Autodesk Inventor part; units mm, degrees
ref_plane "YZ Plane" through (0, 0, 0) normal (1, 0, 0) x (0, 1, 0)
ref_plane "XZ Plane" through (0, 0, 0) normal (0, 1, 0) x (-1, 0, 0)
ref_plane "XY Plane" through (0, 0, 0) normal (0, 0, 1) x (1, 0, 0)
sketch "Sketch1" plane through (0, 0, 0) normal (0, 1, 0) x (-1, 0, 0)
  circle A0 centre (0, 0) radius 17.1346
extrude "Extrusion1" add sketch "Sketch1" along normal blind 10
sketch "Sketch2" plane through (0, 0, 0) normal (0, -1, 0) x (1, 0, 0)
  circle A0 centre (0, 0) radius 14.2353
extrude "Extrusion2" add sketch "Sketch2" along normal blind 5
chamfer "Chamfer1" distance 2 angle 45 1 edges at (-14.2353, -5, 0)
properties part number "Tapon externo"
For this review, take the finished solid that the model builds, in its own axes (mm). A direction names the side the tool comes from. Coordinates: 2 decimals unless noted, no trailing zeros. Order: outer loops, then holes, each group sorted by start corner. A loop starts at its lowest first (then second) coordinate and runs counter-clockwise, first axis right, second up. Notation, with made-up numbers: (46.5, 25.25) -> (57.5, 25.25) arc R27 ccw to (57.5, 43.25) -> close; hole circle Ø7 at (21, -9.5). An arc over 180 degrees is marked (long way). Use CSV: the item, a comma, the result in double quotes. Start each with the question number.
Item 1: For faces 1 (the face through (4, 0, 14)), 2 (the face through (-16.343, 4.93, -5.147)), list the 3-axis set-ups (+Z, -Z, +X, -X, +Y, -Y) from which the entire face can be reached by the end or side of a thin tool; tool diameter is ignored.
Item 2: We need section A-A, the plane x = 0. Give the boundary of the cut face in (y, z).
Item 3: We need section D-D, the plane y = -2. Give the boundary of the cut face in (x, z), then the cut area to 3 significant figures.
Item 4: Insertion check: pin 1 (5 mm diameter, centred on y = 4.5, z = -11, fed in from -X); pin 2 (3 mm diameter, centred on y = 3, z = 12.5, fed in from +X); pin 3 (1 mm diameter, centred on y = 2, z = 9.5, fed in from -X). Each pin has a flat end and moves straight along its axis. Give the tip position at first contact, or say it passes through.
Item 5: We need section B-B, the plane z = 0. Give the boundary of the cut face in (x, y), then the cut area to 3 significant figures.
Item 6: We need section C-C, the plane y = 5.5. Give the boundary of the cut face in (x, z), then the cut area to 3 significant figures.
Item 7: Wall thickness on probe 1 along Y at (x, z) = (12.5, -11.5); probe 2 along Z at (x, y) = (-14, 6.75); probe 3 along Z at (x, y) = (15, 7): over which ranges is each line inside the solid? List them lowest first.
Derived:
1,face 1,"-Y"
1,face 2,"+Y, -Y"
2,outline,"(-5, -12.24) -> (-3, -14.24) -> (0, -14.24) -> (0, -17.13) -> (10, -17.13) -> (10, 17.13) -> (0, 17.13) -> (0, 14.24) -> (-3, 14.24) -> (-5, 12.24) -> close"
3,outline,"circle Ø28.47 at (0, 0)"
3,area,"637 mm^2"
4,pin 1,"stops at x = -14.88"
4,pin 2,"stops at x = 13.14"
4,pin 3,"stops at x = -14.58"
5,outline,"(-17.13, 0) -> (-14.24, 0) -> (-14.24, -3) -> (-12.24, -5) -> (12.24, -5) -> (14.24, -3) -> (14.24, 0) -> (17.13, 0) -> (17.13, 10) -> (-17.13, 10) -> close"
5,area,"481 mm^2"
6,outline,"circle Ø34.27 at (0, 0)"
6,area,"922 mm^2"
7,probe 1,"y = 0 to 10"
7,probe 2,"z = -9.88 to 9.88"
7,probe 3,"z = -8.28 to 8.28"
